```python
from build123d import *

# Parameters (mm, degrees)
SKETCH1_W           = 150
SKETCH1_H           = 80
BOSS_EXTRUDE1_DEPTH = 7
SKETCH2_W           = 6
SKETCH2_H           = 40
CUT_EXTRUDE2_DEPTH  = 7
SKETCH3_R           = 25
CUT_EXTRUDE3_DEPTH  = 7
CUT_EXTRUDE5_DEPTH  = 7
CUT_EXTRUDE6_DEPTH  = 7
SKETCH6_R           = 2.5
CUT_EXTRUDE7_DEPTH  = 7
BOSS_EXTRUDE2_DEPTH = 6
CUT_EXTRUDE8_DEPTH  = 6
SKETCH10_W          = 6
SKETCH10_H          = 20
BOSS_EXTRUDE3_DEPTH = 13
CUT_EXTRUDE9_DEPTH  = 13
SKETCH12_R          = 2.5
CUT_EXTRUDE10_DEPTH = 13
BOSS_EXTRUDE5_DEPTH = 5
SKETCH14_R          = 2
CUT_EXTRUDE11_DEPTH = 20.091883092
CUT_EXTRUDE13_DEPTH = 6
BOSS_EXTRUDE6_DEPTH = 7


with BuildPart() as part:
    # Sketch1 → Boss-Extrude1 (new body)
    with BuildSketch(Plane.XY):
        with Locations((75, 40)):
            Rectangle(SKETCH1_W, SKETCH1_H)
    extrude(amount=BOSS_EXTRUDE1_DEPTH)

    # Sketch2 → Cut-Extrude2 (cut)
    with BuildSketch(Plane.XY.offset(7)):
        with Locations((3, 40)):
            Rectangle(SKETCH2_W, SKETCH2_H)
    extrude(amount=-CUT_EXTRUDE2_DEPTH, mode=Mode.SUBTRACT)

    # Sketch3 → Cut-Extrude3 (cut)
    with BuildSketch(Plane.XY.offset(7)):
        with Locations((65, 40)):
            Circle(SKETCH3_R)
    extrude(amount=-CUT_EXTRUDE3_DEPTH, mode=Mode.SUBTRACT)

    # Sketch4 → Cut-Extrude5 (cut)
    with BuildSketch(Plane.XY.offset(7)):
        with BuildLine():
            Line((15.828446624, 69.975175599), (15.828446624, 10.024824401))
            Line((15.828446624, 10.024824401), (36.358795003, 10.024824401))
            Line((36.358795003, 10.024824401), (36.358795003, 15.793980576))
            ThreePointArc((36.358795003, 15.793980576), (27.5, 40), (36.358795003, 64.206019424))
            Line((36.358795003, 64.206019424), (36.358795003, 69.975175599))
            Line((36.358795003, 69.975175599), (15.828446624, 69.975175599))
        make_face()
    extrude(amount=-CUT_EXTRUDE5_DEPTH, mode=Mode.SUBTRACT)

    # Sketch5 → Cut-Extrude6 (cut)
    with BuildSketch(Plane.XY.offset(7)):
        with BuildLine():
            Line((93.631196157, 69.975175599), (93.631196157, 64.217857185))
            ThreePointArc((93.631196157, 64.217857185), (102.5, 40), (93.631196157, 15.782142815))
            Line((93.631196157, 15.782142815), (93.631196157, 10.024824401))
            Line((93.631196157, 10.024824401), (137.533061217, 10.024824401))
            Line((137.533061217, 10.024824401), (137.533061217, 69.975175599))
            Line((137.533061217, 69.975175599), (93.631196157, 69.975175599))
        make_face()
    extrude(amount=-CUT_EXTRUDE6_DEPTH, mode=Mode.SUBTRACT)

    # Sketch6 → Cut-Extrude7 (cut)
    with BuildSketch(Plane.XY.offset(7)):
        with Locations((97, 40)):
            Circle(SKETCH6_R)
        with Locations((87.627416998, 17.372583002)):
            Circle(SKETCH6_R)
        with Locations((65, 8)):
            Circle(SKETCH6_R)
        with Locations((42.372583002, 17.372583002)):
            Circle(SKETCH6_R)
        with Locations((33, 40)):
            Circle(SKETCH6_R)
        with Locations((42.372583002, 62.627416998)):
            Circle(SKETCH6_R)
        with Locations((65, 72)):
            Circle(SKETCH6_R)
        with Locations((87.627416998, 62.627416998)):
            Circle(SKETCH6_R)
    extrude(amount=-CUT_EXTRUDE7_DEPTH, mode=Mode.SUBTRACT)

    # Sketch8 → Boss-Extrude2 (add)
    with BuildSketch(Plane.ZY):
        Polygon((0, 60), (-20, 80), (0, 80), align=None)
    extrude(amount=-BOSS_EXTRUDE2_DEPTH)

    # Sketch9 → Cut-Extrude8 (cut)
    with BuildSketch(Plane.ZY):
        Polygon((-13, 80), (-13, 73), (-20, 80), align=None)
    extrude(amount=-CUT_EXTRUDE8_DEPTH, mode=Mode.SUBTRACT)

    # Sketch10 → Boss-Extrude3 (add)
    with BuildSketch(Plane(origin=(0, 0, 0), x_dir=(-1, 0, 0), z_dir=(0, 0, -1))):
        with Locations((-3, 10)):
            Rectangle(SKETCH10_W, SKETCH10_H)
    extrude(amount=BOSS_EXTRUDE3_DEPTH)

    # Sketch11 → Cut-Extrude9 (cut)
    with BuildSketch(Plane.ZY):
        Polygon((0, 20), (-13, 7), (-13, 20), align=None)
    extrude(amount=-CUT_EXTRUDE9_DEPTH, mode=Mode.SUBTRACT)

    # Sketch12 → Cut-Extrude10 (cut)
    with BuildSketch(Plane.XY.offset(7)):
        with Locations((130, 75)):
            Circle(SKETCH12_R)
        with Locations((115, 75)):
            Circle(SKETCH12_R)
        with Locations((130, 5)):
            Circle(SKETCH12_R)
        with Locations((115, 5)):
            Circle(SKETCH12_R)
    extrude(amount=-CUT_EXTRUDE10_DEPTH, mode=Mode.SUBTRACT)

    # Sketch13 → Boss-Extrude5 (add)
    with BuildSketch(Plane(origin=(6, 0, 0), x_dir=(0, 0, -1), z_dir=(1, 0, 0))):
        Polygon((0, 60), (13, 73), (13, 80), (0, 80), align=None)
        Polygon((13, 0), (0, 0), (0, 20), (13, 7), align=None)
    extrude(amount=BOSS_EXTRUDE5_DEPTH)

    # Sketch14 → Cut-Extrude11 (cut, through all)
    with BuildSketch(Plane(origin=(0, 30, 30), x_dir=(1, 0, 0), z_dir=(0, -0.707106781, -0.707106781))):
        with Locations((3, -47.618795027)):
            Circle(SKETCH14_R)
        with Locations((3, -55.618795027)):
            Circle(SKETCH14_R)
    cut_extrude11 = extrude(amount=-CUT_EXTRUDE11_DEPTH, mode=Mode.SUBTRACT)

    # Sketch15 → Cut-Extrude13 (cut)
    with BuildSketch(Plane.ZY):
        Polygon((7, 70), (-3, 80), (7, 80), align=None)
        Polygon((-3, 0), (7, 0), (7, 10), align=None)
    extrude(amount=-CUT_EXTRUDE13_DEPTH, mode=Mode.SUBTRACT)

    # Mirror1: Cut-Extrude11 across plane
    add(cut_extrude11.mirror(Plane(origin=(0, 40, 0), x_dir=(0, 0, 1), z_dir=(0, -1, 0))), mode=Mode.SUBTRACT)

    # Sketch17 → Boss-Extrude6 (add)
    with BuildSketch(Plane.XY.offset(7)):
        Polygon((150, 80), (175, 65.56624327), (175, 14.43375673), (150, 0), align=None)
    extrude(amount=-BOSS_EXTRUDE6_DEPTH)


solid = part.part
```
Check sheet for the modelled part. Datum: model origin and axes. Units: mm. A direction names the side the tool comes from. Give positions to 0.01 mm unless a question says otherwise; leave off trailing zeros. Order: outer loops, then holes, each group sorted by start corner. A loop starts at its lowest first (then second) coordinate and runs counter-clockwise, first axis right, second up. Notation, with made-up numbers: M 70.5,12.5 L 106.5,12.5 A27 ccw 106.5,48.5 Z; hole C -17.75,19.25 d8. An arc over 180 degrees is marked long. Answer in a Markdown table with one row per item.
1) Access from +Z, -Z, +X, -X, +Y, -Y to the whole of each face (thin tool, end or side, straight path). Record for faces 1 (the flat face through (93.631, 67, 4)), 2 (the cylindrical face through (1.41, 11.28, -0.34)), 3 (the flat face through (5, 66, -6)), 4 (the flat face through (11, 72, -5)).
Filled sheet:
| item | result |
|---|---|
| face 1 | +Z, -Z |
| face 2 | none |
| face 3 | -Z, +X, -X |
| face 4 | -Z, +X, +Y, -Y |
2) Cross-section at B-B, the plane y = 40. Enter the section's corners in (x, z).
Filled sheet:
| item | result |
|---|---|
| outline | M 6,0 L 15.83,0 L 15.83,7 L 6,7 Z; M 27.5,0 L 30.5,0 L 30.5,7 L 27.5,7 Z; M 35.5,0 L 40,0 L 40,7 L 35.5,7 Z; M 90,0 L 94.5,0 L 94.5,7 L 90,7 Z; M 99.5,0 L 102.5,0 L 102.5,7 L 99.5,7 Z; M 137.53,0 L 175,0 L 175,7 L 137.53,7 Z |
3) Cross-section at C-C, the plane y = 28. Enter the section's corners in (x, z).
Filled sheet:
| item | result |
|---|---|
| outline | M 6,0 L 15.83,0 L 15.83,7 L 6,7 Z; M 29.47,0 L 43.07,0 L 43.07,7 L 29.47,7 Z; M 86.93,0 L 100.53,0 L 100.53,7 L 86.93,7 Z; M 137.53,0 L 175,0 L 175,7 L 137.53,7 Z |
4) Release check for a two-part mould opening along Y. For faces 5 (the flat face through (0, 70, -3)), 6 (the flat face through (36.359, 13, 4)), 7 (the flat face through (59, 0, 2)) record: +Y half, -Y half, draft (parallel to the pull), parting line (faces both ways), or undercut.
Filled sheet:
| item | result |
|---|---|
| face 5 | draft |
| face 6 | undercut |
| face 7 | -Y half |
5) Cross-section at A-A, the plane x = 65. Enter the section's corners in (y, z).
Filled sheet:
| item | result |
|---|---|
| outline | M 0,0 L 5.5,0 L 5.5,7 L 0,7 Z; M 10.5,0 L 15,0 L 15,7 L 10.5,7 Z; M 65,0 L 69.5,0 L 69.5,7 L 65,7 Z; M 74.5,0 L 80,0 L 80,7 L 74.5,7 Z |
6) Gauge pin test, flat ends, axial feed: P1, Ø6, axis at y = 30, z = 4, coming from the -X side; P2, Ø3, axis at x = 130, y = 5, coming from the -Z side; P3, Ø6.5, axis at x = 33, y = 40, coming from the -Z side; P4, Ø1.8, axis at x = 2.5, z = 3.5, coming from the +Y side. Record the tip position at first contact, or that the pin passes through.
Filled sheet:
| item | result |
|---|---|
| P1 | stops at x = 6 |
| P2 | passes through |
| P3 | stops at z = 0 |
| P4 | stops at y = 74.4 |
7) Cross-section at D-D, the plane x = 146. Enter the section's corners in (y, z).
Filled sheet:
| item | result |
|---|---|
| outline | M 0,0 L 80,0 L 80,7 L 0,7 Z |
8) Thickness scan on L1, parallel to Y at x = 130, z = 4.75; L2, parallel to Y at x = 65, z = 2.75; L3, parallel to X at y = 55.5, z = 3.25. Record the ranges inside material, lowest first. Write a range as [from, to].
Filled sheet:
| item | result |
|---|---|
| L1 | y = [0, 2.5], [7.5, 10.02], [69.98, 72.5], [77.5, 80] |
| L2 | y = [0, 5.5], [10.5, 15], [65, 69.5], [74.5, 80] |
| L3 | x = [6, 15.83], [30.85, 45.38], [84.62, 99.15], [137.53, 175] |
